For this review, take the finished solid that the model builds, in its own axes (mm). Face numbers are marked on the shaded views. A direction names the side the tool comes from. Coordinates: 2 decimals unless noted, no trailing zeros. Write each loop counter-clockwise with the first axis right and the second up, starting at its lowest first coordinate (ties: lowest second). Pieces come first, ordered by that corner, then holes. Notation, with made-up numbers: (6, -9) -> (65, -9) arc R7 ccw to (65, -5) -> close; hole circle Ø10 at (-17.75, 17.25). An arc over 180 degrees is marked (long way). One line per item, written item: value. Start each with the question number.
1) Add section B-B (z = 6.25). State the section outline as (x, y) points, and give its area (3 significant figures).
2) For pin 1 Ø13 at (x, y) = (-13, -4.5) entering from +Z; pin 2 Ø4 at (y, z) = (0, 10) entering from -X, all flat-tipped, find the tip position at first contact; note any pin that passes through.
3) Add section C-C (x = -43.5). State the section outline as (y, z) points.
4) Machinability: for the marked faces 1 and 2, which of the approach directions +Z, -Z, +X, -X, +Y, -Y give a long, thin tool a straight path to every point of the face, cutting with its end or side? Answer none if there is none.
5) Add section D-D (y = -12). State the section outline as (x, z) points.
6) Mouldability with a two-part tool opening along Y and no side actions: class the marked faces 3, 4, 5 and 6 as released by +Y, released by -Y, zero draft, split by the parting line, or undercut.
7) For probe 1 along X at (y, z) = (19, 8.25); probe 2 along Y at (x, z) = (31, 14.75); probe 3 along X at (y, z) = (-9.5, 17.25), list the stretches that pass through material, from the lowest coordinate up. Write a range as from..to.
8) Add section A-A (y = 0). State the section outline as (x, z) points, and give its area (3 significant figures).
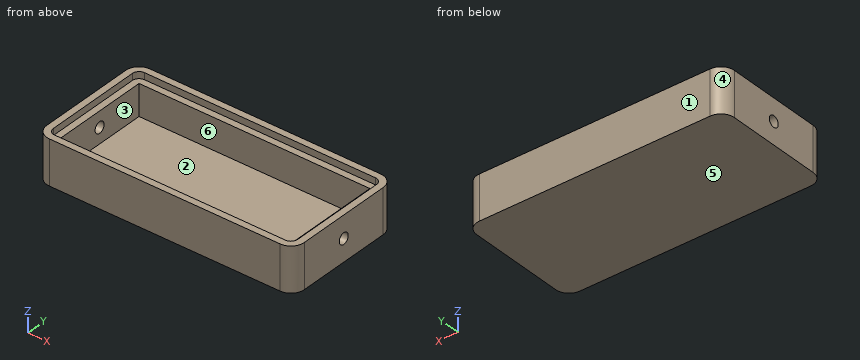
from build123d import *

# Parameters (mm, degrees)
ESQUISSE1_W             = 116
ESQUISSE1_H             = 56
BOSS_EXTRU_1_DEPTH      = 20
CONG_1_R                = 6
COQUE1_T                = -3
ESQUISSE2_W             = 104
ESQUISSE2_H             = 44
BOSS_EXTRU_2_DEPTH      = 14
ESQUISSE3_R             = 2.5
ENL_V_MAT_EXTRU_1_DEPTH = 121.995867698


with BuildPart() as part:
    # Esquisse1 → Boss.-Extru.1 (new body)
    with BuildSketch(Plane.XY):
        Rectangle(ESQUISSE1_W, ESQUISSE1_H)
    extrude(amount=BOSS_EXTRU_1_DEPTH)

    # Congé1
    cong_1_edges = [part.edges().sort_by_distance(p)[0] for p in [
        (58, -28, 10),
        (-58, -28, 10),
        (-58, 28, 10),
        (58, 28, 10),
    ]]
    fillet(cong_1_edges, radius=CONG_1_R)

    # Coque1
    coque1_openings = [part.faces().sort_by_distance(p)[0] for p in [
        (0, 0, 20),
    ]]
    offset(amount=COQUE1_T, openings=coque1_openings, kind=Kind.INTERSECTION)

    # Esquisse2 → Boss.-Extru.2 (add)
    with BuildSketch(Plane.XY.offset(3)):
        with BuildLine():
            Line((52, 25), (-52, 25))
            ThreePointArc((-52, 25), (-54.121320344, 24.121320344), (-55, 22))
            Line((-55, 22), (-55, -22))
            ThreePointArc((-55, -22), (-54.121320344, -24.121320344), (-52, -25))
            Line((-52, -25), (52, -25))
            ThreePointArc((52, -25), (54.121320344, -24.121320344), (55, -22))
            Line((55, -22), (55, 22))
            ThreePointArc((55, 22), (54.121320344, 24.121320344), (52, 25))
        make_face()
        Rectangle(ESQUISSE2_W, ESQUISSE2_H, mode=Mode.SUBTRACT)
    extrude(amount=BOSS_EXTRU_2_DEPTH)

    # Esquisse3 → Enlèv. mat.-Extru.1 (cut, through all)
    with BuildSketch(Plane.ZY.offset(58)):
        with Locations((10, 0)):
            Circle(ESQUISSE3_R)
    extrude(amount=-ENL_V_MAT_EXTRU_1_DEPTH, mode=Mode.SUBTRACT)


solid = part.part
Numbers:
1. outline: (-58, -22) arc R6 ccw to (-52, -28) -> (52, -28) arc R6 ccw to (58, -22) -> (58, 22) arc R6 ccw to (52, 28) -> (-52, 28) arc R6 ccw to (-58, 22) -> close; hole (-52, -22) -> (52, -22) -> (52, 22) -> (-52, 22) -> close
1. area: 1,890 mm²
2. pin 1: z = 3
2. pin 2: through
3. outline: (-28, 0) -> (28, 0) -> (28, 20) -> (25, 20) -> (25, 17) -> (22, 17) -> (22, 3) -> (-22, 3) -> (-22, 17) -> (-25, 17) -> (-25, 20) -> (-28, 20) -> close
4. face 1: +Z, -Z, +X, -X, +Y
4. face 2: +Z
5. outline: (-58, 0) -> (58, 0) -> (58, 20) -> (55, 20) -> (55, 17) -> (52, 17) -> (52, 3) -> (-52, 3) -> (-52, 17) -> (-55, 17) -> (-55, 20) -> (-58, 20) -> close
6. face 3: undercut
6. face 4: released by +Y
6. face 5: zero draft
6. face 6: undercut
7. probe 1: -58..-52, 52..58
7. probe 2: -28..-22, 22..28
7. probe 3: -58..-55, 55..58
8. outline: (-58, 0) -> (58, 0) -> (58, 7.5) -> (52, 7.5) -> (52, 3) -> (-52, 3) -> (-52, 7.5) -> (-58, 7.5) -> close; (-58, 12.5) -> (-52, 12.5) -> (-52, 17) -> (-55, 17) -> (-55, 20) -> (-58, 20) -> close; (52, 12.5) -> (58, 12.5) -> (58, 20) -> (55, 20) -> (55, 17) -> (52, 17) -> close
8. area: 474 mm²
